Geometry check sheet. Reference: the model listing, model coordinates, mm. A direction names the side the tool comes from. Round coordinates to 2 decimals unless told otherwise and drop trailing zeros. Loops run counter-clockwise (first coordinate to the right, second up) from the corner with the lowest first, then second, coordinate; pieces in that order, holes last.
```python
from build123d import *

# Parameters (mm, degrees)
BOSS_EXTRUDE1_DEPTH            = 6.35
F_3_16_0_1875_DIAMETER_HOLE1_D = 4.7625
F_21_0_159_DIAMETER_HOLE1_D    = 4.0386
SKETCH4_W                      = 15.875
SKETCH4_H                      = 12.7
CUT_EXTRUDE1_DEPTH             = 3.175


with BuildPart() as part:
    # Sketch1 → Boss-Extrude1 (new body)
    with BuildSketch(Plane(origin=(0, 0, 0), x_dir=(1, 0, 0), z_dir=(0, 1, 0))):
        with BuildLine():
            Line((-63.5, 6.35), (63.5, 6.35))
            ThreePointArc((63.5, 6.35), (69.85, 0), (63.5, -6.35))
            Line((63.5, -6.35), (-63.5, -6.35))
            ThreePointArc((-63.5, -6.35), (-69.85, 0), (-63.5, 6.35))
        make_face()
    extrude(amount=BOSS_EXTRUDE1_DEPTH)

    # 3/16 (0.1875) Diameter Hole1 (through all)
    with Locations(Plane(origin=(0, 6.35, 0), x_dir=(1, 0, 0), z_dir=(0, 1, 0))):
        with Locations((-63.5, 0)):
            Hole(F_3_16_0_1875_DIAMETER_HOLE1_D / 2)

    # #21 (0.159) Diameter Hole1 (through all)
    with Locations(Plane(origin=(0, 6.35, 0), x_dir=(1, 0, 0), z_dir=(0, 1, 0))):
        with Locations((63.5, 0)):
            Hole(F_21_0_159_DIAMETER_HOLE1_D / 2)

    # Sketch4 → Cut-Extrude1 (cut)
    with BuildSketch(Plane(origin=(0, 6.35, 0), x_dir=(1, 0, 0), z_dir=(0, 1, 0))):
        with Locations((63.5, 0)):
            Rectangle(SKETCH4_W, SKETCH4_H)
    extrude(amount=-CUT_EXTRUDE1_DEPTH, mode=Mode.SUBTRACT)


solid = part.part
```
1) Sectioned sample at A-A, the plane z = 0. State how many separate pieces and enclosed holes the cut face has, then the cut area to 3 significant figures.
Report:
separate pieces: 3
enclosed holes: 0
area: 799 mm2
2) Scan lines: line 1 along Z through (x, y) = (-63.5, 3.25); line 2 along Z through (x, y) = (63.5, 1.15); line 3 along Y through (x, z) = (62.5, 5) (3 decimals). Record each from-to range of solid material in increasing order.
Report:
line 1: z = -6.35 to -2.38, 2.38 to 6.35
line 2: z = -6.35 to -2.02, 2.02 to 6.35
line 3: y = 0 to 3.175
3) Sectioned sample at B-B, the plane y = 4.25. Record the cut outline in (x, z), then the cut area to 3 significant figures.
Report:
outline: (-63.5, -6.35) - (55.56, -6.35) - (55.56, 6.35) - (-63.5, 6.35) arc R6.35 ccw to start; hole circle Ø4.76 at (-63.5, 0)
area: 1,560 mm2
4) Mould release check, pull along Z, two halves, no side actions. Record for faces 3 (the face through (65.517, 1.565, -0.089)), 4 (the face through (69.85, 1.57, -0.14)), 5 (the face through (55.562, 5, 0)): +Z half, -Z half, draft (parallel to the pull), parting line (faces both ways), or undercut.
Report:
face 3: undercut
face 4: parting line
face 5: draft
5) Gauge pin test, flat ends, axial feed: pin 1 (3 mm diameter, centred on y = 1.5, z = -4.5, fed in from -X); pin 2 (4 mm diameter, centred on x = -31, z = -2.5, fed in from -Y); pin 3 (1.5 mm diameter, centred on y = 5.5, z = 4.5, fed in from +X); pin 4 (3.5 mm diameter, centred on x = 63.5, z = 0, fed in from +Y). Record the tip position at first contact, or that the pin passes through.
Report:
pin 1: stops at x = -69.1
pin 2: stops at y = 0
pin 3: stops at x = 55.56
pin 4: passes through
6) Access from +Z, -Z, +X, -X, +Y, -Y to the whole of each face (thin tool, end or side, straight path). Record for faces 1 (the face through (61, 3.175, 0)), 2 (the face through (-6, 6.35, 0)).
Report:
face 1: +Z, -Z, +X, +Y
face 2: +Z, -Z, +X, -X, +Y
